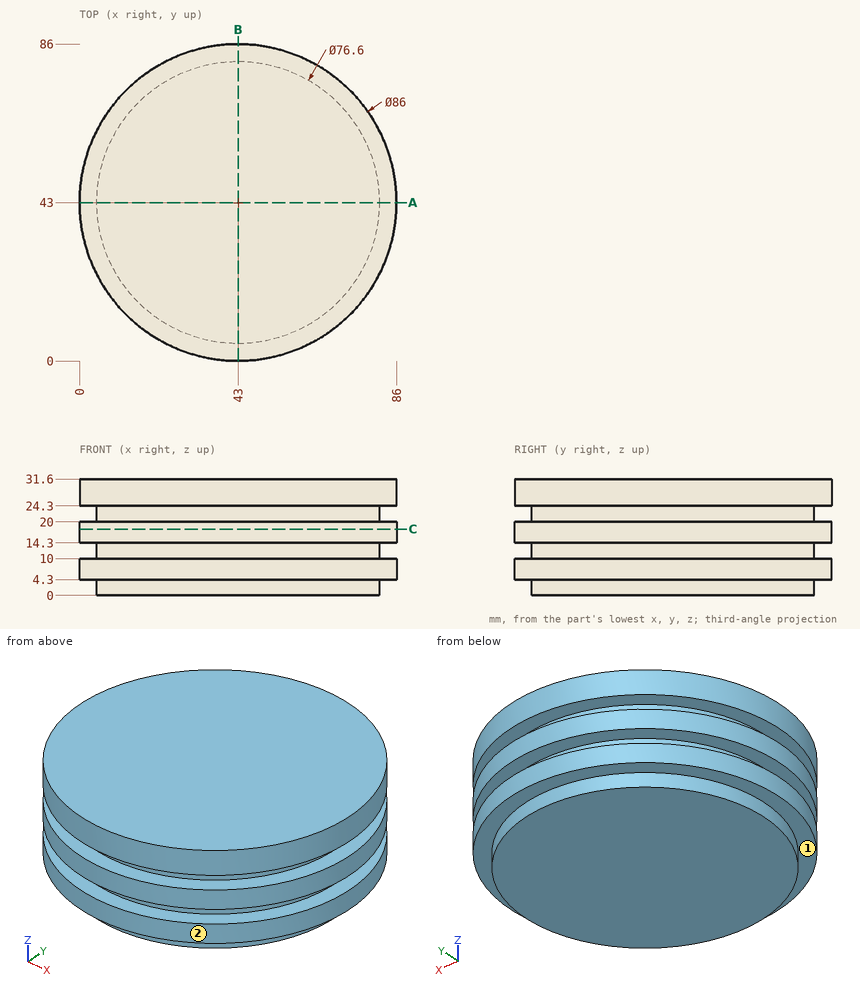
Geometry check sheet. Reference: drawing and pictorial views, mm from the part's lowest x, y, z. Give positions to 0.01 mm unless a question says otherwise; leave off trailing zeros. Order: outer loops, then holes, each group sorted by start corner. A loop starts at its lowest first (then second) coordinate and runs counter-clockwise, first axis right, second up. Notation, with made-up numbers: (53, -39.5) -> (58, -39.5) arc R21 ccw to (58, -30.5) -> close; hole circle Ø9 at (-22.5, 76.25). An arc over 180 degrees is marked (long way). Use CSV: the item, a comma, the result in double quotes. Start each with the question number.
1) Mould release check, pull along X, two halves, no side actions. Record for the marked faces 1 and 2: released by +X, released by -X, zero draft, split by the parting line, or undercut.
2) Sectioned sample at A-A, the plane y = 43. Record the boundary of the cut face in (x, z), plus the area to 3 significant figures.
3) Sectioned sample at C-C, the plane z = 18. Record the boundary of the cut face in (x, y).
4) Go/stop test with flat-tipped pins: P1, Ø10, axis at x = 45, y = 8.5, coming from the -Z side; P2, Ø8, axis at x = 41.5, z = 19.5, coming from the -Y side; P3, Ø8, axis at y = 18.5, z = 17, coming from the -X side; P4, Ø12, axis at y = 26, z = 15.5, coming from the -X side. Record where each tip stops, or that it passes through.
5) Material ranges on line 1 (Z direction, x = 57.5, y = 81.5); line 2 (X direction, y = 43.5, z = 10.5); line 3 (X direction, y = 44.5, z = 17), recorded low to high. Write a range as from..to.
Recorded:
1,face 1,"zero draft"
1,face 2,"split by the parting line"
2,outline,"(0, 4.3) -> (4.7, 4.3) -> (4.7, 0) -> (81.3, 0) -> (81.3, 4.3) -> (86, 4.3) -> (86, 10) -> (81.3, 10) -> (81.3, 14.3) -> (86, 14.3) -> (86, 20) -> (81.3, 20) -> (81.3, 24.3) -> (86, 24.3) -> (86, 31.6) -> (0, 31.6) -> (0, 24.3) -> (4.7, 24.3) -> (4.7, 20) -> (0, 20) -> (0, 14.3) -> (4.7, 14.3) -> (4.7, 10) -> (0, 10) -> close"
2,area,"2,600 mm2"
3,outline,"circle Ø86 at (43, 43)"
4,P1,"z = 0"
4,P2,"y = 0"
4,P3,"x = 5.2"
4,P4,"x = 1.43"
5,line 1,"4.3..10, 14.3..20, 24.3..31.6"
5,line 2,"4.7..81.3"
5,line 3,"0.03..85.97"
